Model file for the job. Use its own axes, mm. Give positions to 0.01 mm unless a question says otherwise; leave off trailing zeros. Loops run counter-clockwise (first coordinate to the right, second up) from the corner with the lowest first, then second, coordinate; pieces in that order, holes last. Notation, with made-up numbers: M -7.75,20.25 L 7.25,20.25 A25 ccw 7.25,34.25 Z; hole C -37.75,76.25 d6. An arc over 180 degrees is marked long. Answer in a Markdown table with one row per item.
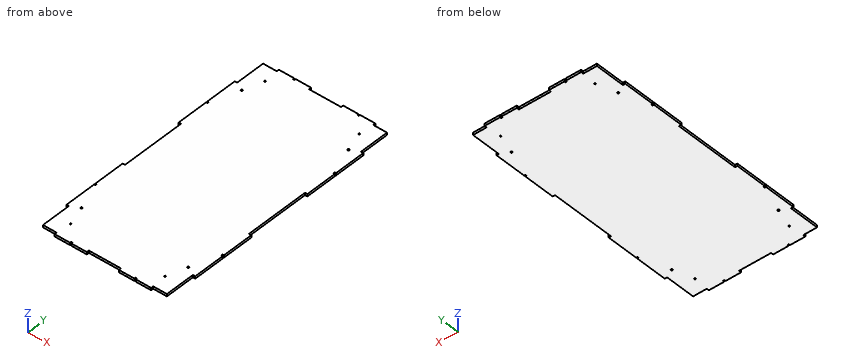
```python
from build123d import *

# Parameters (mm, degrees)
BOSS_EXTRUDE1_DEPTH     = 5.5
CUT_EXTRUDE1_DEPTH      = 664.465030112
CUT_EXTRUDE1_DEPTH_BACK = 664.465030112
SKETCH3_R               = 1.6
CUT_EXTRUDE2_DEPTH      = 664.465030112


with BuildPart() as part:
    # Sketch1 → Boss-Extrude1 (new body)
    with BuildSketch(Plane.XY):
        Polygon((-0.002685186, 588.997205838), (-0.002685186, 519.497205838), (-5.502685186, 519.497205838), (-5.502685186, 446.122205838), (-2.252685186, 446.122205838), (-2.252685186, 444.497205838), (-2.252685186, 442.872205838), (-5.502685186, 442.872205838), (-5.502685186, 369.497205838), (-0.002685186, 369.497205838), (-0.002685186, 219.497205838), (-5.502685186, 219.497205838), (-5.502685186, 146.122205838), (-2.252685186, 146.122205838), (-2.252685186, 144.497205838), (-2.252685186, 142.872205838), (-5.502685186, 142.872205838), (-5.502685186, 69.497205838), (-0.002685186, 69.497205838), (-0.002685186, -0.002794162), (31.997314814, -0.002794162), (31.997314814, -5.502794162), (67.872314814, -5.502794162), (67.872314814, -2.252794162), (69.497314814, -2.252794162), (71.122314814, -2.252794162), (71.122314814, -5.502794162), (106.997314814, -5.502794162), (106.997314814, -0.002794162), (181.997314814, -0.002794162), (181.997314814, -5.502794162), (217.872314814, -5.502794162), (217.872314814, -2.252794162), (219.497314814, -2.252794162), (221.122314814, -2.252794162), (221.122314814, -5.502794162), (256.997314814, -5.502794162), (256.997314814, -0.002794162), (288.997314814, -0.002794162), (288.997314814, 69.497205838), (294.497314814, 69.497205838), (294.497314814, 142.872205838), (291.247314814, 142.872205838), (291.247314814, 144.497205838), (291.247314814, 146.122205838), (294.497314814, 146.122205838), (294.497314814, 219.497205838), (288.997314814, 219.497205838), (288.997314814, 369.497205838), (294.497314814, 369.497205838), (294.497314814, 442.872205838), (291.247314814, 442.872205838), (291.247314814, 444.497205838), (291.247314814, 446.122205838), (294.497314814, 446.122205838), (294.497314814, 519.497205838), (288.997314814, 519.497205838), (288.997314814, 588.997205838), (256.997314814, 588.997205838), (256.997314814, 594.497205838), (221.122314814, 594.497205838), (221.122314814, 591.247205838), (219.497314814, 591.247205838), (217.872314814, 591.247205838), (217.872314814, 594.497205838), (181.997314814, 594.497205838), (181.997314814, 588.997205838), (106.997314814, 588.997205838), (106.997314814, 594.497205838), (71.122314814, 594.497205838), (71.122314814, 591.247205838), (69.497314814, 591.247205838), (67.872314814, 591.247205838), (67.872314814, 594.497205838), (31.997314814, 594.497205838), (31.997314814, 588.997205838), align=None)
    extrude(amount=BOSS_EXTRUDE1_DEPTH)

    # Sketch2 → Cut-Extrude1 (cut, two sides: drawn at the far end of the back side and taken through both)
    with BuildSketch(Plane.XY.offset(-CUT_EXTRUDE1_DEPTH_BACK)):
        with BuildLine():
            ThreePointArc((270.997314814, 508.997205838), (268.997314814, 510.997205838), (266.997314814, 508.997205838))
            Line((266.997314814, 508.997205838), (268.997314814, 508.997205838))
            Line((268.997314814, 508.997205838), (268.997314814, 506.997205838))
            ThreePointArc((268.997314814, 506.997205838), (270.411528376, 507.582992276), (270.997314814, 508.997205838))
        make_face()
        with BuildLine():
            Line((268.997314814, 508.997205838), (266.997314814, 508.997205838))
            ThreePointArc((266.997314814, 508.997205838), (267.583101251, 507.582992276), (268.997314814, 506.997205838))
            Line((268.997314814, 506.997205838), (268.997314814, 508.997205838))
        make_face()
        with BuildLine():
            Line((19.997314814, 506.997205838), (19.997314814, 508.997205838))
            Line((19.997314814, 508.997205838), (21.997314814, 508.997205838))
            ThreePointArc((21.997314814, 508.997205838), (18.583101251, 510.4114194), (19.997314814, 506.997205838))
        make_face()
        with BuildLine():
            Line((21.997314814, 508.997205838), (19.997314814, 508.997205838))
            Line((19.997314814, 508.997205838), (19.997314814, 506.997205838))
            ThreePointArc((19.997314814, 506.997205838), (21.411528376, 507.582992276), (21.997314814, 508.997205838))
        make_face()
        with BuildLine():
            ThreePointArc((21.997314814, 79.997205838), (21.411528376, 81.4114194), (19.997314814, 81.997205838))
            Line((19.997314814, 81.997205838), (19.997314814, 79.997205838))
            Line((19.997314814, 79.997205838), (21.997314814, 79.997205838))
        make_face()
        with BuildLine():
            Line((19.997314814, 79.997205838), (19.997314814, 81.997205838))
            ThreePointArc((19.997314814, 81.997205838), (18.583101251, 78.582992276), (21.997314814, 79.997205838))
            Line((21.997314814, 79.997205838), (19.997314814, 79.997205838))
        make_face()
        with BuildLine():
            ThreePointArc((270.997314814, 79.997205838), (270.411528376, 81.4114194), (268.997314814, 81.997205838))
            Line((268.997314814, 81.997205838), (268.997314814, 79.997205838))
            Line((268.997314814, 79.997205838), (266.997314814, 79.997205838))
            ThreePointArc((266.997314814, 79.997205838), (268.997314814, 77.997205838), (270.997314814, 79.997205838))
        make_face()
        with BuildLine():
            Line((268.997314814, 79.997205838), (268.997314814, 81.997205838))
            ThreePointArc((268.997314814, 81.997205838), (267.583101251, 81.4114194), (266.997314814, 79.997205838))
            Line((266.997314814, 79.997205838), (268.997314814, 79.997205838))
        make_face()
    extrude(amount=CUT_EXTRUDE1_DEPTH + CUT_EXTRUDE1_DEPTH_BACK, mode=Mode.SUBTRACT)

    # Sketch3 → Cut-Extrude2 (cut, through all)
    with BuildSketch(Plane.XY.offset(5.5)):
        with Locations((34.497314814, 554.497205838)):
            Circle(SKETCH3_R)
        with Locations((254.497314814, 554.497205838)):
            Circle(SKETCH3_R)
        with Locations((34.497314814, 34.497205838)):
            Circle(SKETCH3_R)
        with Locations((254.497314814, 34.497205838)):
            Circle(SKETCH3_R)
    extrude(amount=-CUT_EXTRUDE2_DEPTH, mode=Mode.SUBTRACT)


solid = part.part
```
(1) Wall check: L1, parallel to Y at x = 148, z = 4.35; L2, parallel to X at y = 338.5, z = 2.85. Give the ranges that are in metal, low to high.
Established:
| item | result |
|---|---|
| L1 | y = 0 to 589 |
| L2 | x = 0 to 289 |
(2) Flat gauge pins, fed straight in: P1, Ø1.6, axis at x = -2.5, z = 3, coming from the -Y side; P2, Ø1.5, axis at y = 365, z = 2, coming from the +X side; P3, Ø1.9, axis at x = 254.5, y = 554.5, coming from the +Z side; P4, Ø2.5, axis at y = -4.5, z = 1.5, coming from the -X side. Where does each tip first touch, or does it go through?
Established:
| item | result |
|---|---|
| P1 | stops at y = 69.5 |
| P2 | stops at x = 289 |
| P3 | passes through |
| P4 | stops at x = 32 |
(3) Saw through at A-A, the plane y = 227.5. Give the cut face in (x, z).
Established:
| item | result |
|---|---|
| outline | M 0,0 L 289,0 L 289,5.5 L 0,5.5 Z |
(4) Saw through at B-B, the plane x = 164. Give the cut face in (y, z).
Established:
| item | result |
|---|---|
| outline | M 0,0 L 589,0 L 589,5.5 L 0,5.5 Z |
(5) Saw through at C-C, the plane z = 2.75. Count the separate pieces of the cut face and the enclosed holes in it, and give its area (3 significant figures).
Established:
| item | result |
|---|---|
| separate pieces | 1 |
| enclosed holes | 8 |
| area | 175,000 mm2 |
